```python
from build123d import *

# Parameters (mm, degrees)
F0_R     = 4
F0_R_2   = 29.171031
F1_DEPTH = 10


with BuildPart() as f1:
    # F0 (on Front) → F1 (new body)
    with BuildSketch(Plane.XZ):
        with BuildLine():
            Line((200, 125), (-180, 125))
            ThreePointArc((-180, 125), (-194.142136, 119.142136), (-200, 105))
            Line((-200, 105), (-200, -45))
            ThreePointArc((-200, -45), (-143.431458, -68.431458), (-120, -125))
            Line((-120, -125), (200, -125))
            Line((200, -125), (200, 125))
        make_face()
        with Locations((-55.033423, -4.654916)):
            Circle(F0_R, mode=Mode.SUBTRACT)
        with Locations((5.235739, -4.654916)):
            Circle(F0_R, mode=Mode.SUBTRACT)
        with Locations((66.157822, -4.654916)):
            Circle(F0_R, mode=Mode.SUBTRACT)
        with Locations((118.3732, -4.654916)):
            Circle(F0_R, mode=Mode.SUBTRACT)
        with Locations((160.996102, -4.654916)):
            Circle(F0_R, mode=Mode.SUBTRACT)
        with Locations((-150.960162, 44.787358)):
            Circle(F0_R_2, mode=Mode.SUBTRACT)
        with Locations((-59.337278, 45.036767)):
            Circle(F0_R, mode=Mode.SUBTRACT)
        with Locations((-60.269162, 95.248777)):
            Circle(F0_R, mode=Mode.SUBTRACT)
        with Locations((0.931884, 45.036767)):
            Circle(F0_R, mode=Mode.SUBTRACT)
        with Locations((61.853966, 45.036767)):
            Circle(F0_R, mode=Mode.SUBTRACT)
        with Locations((114.069345, 45.036767)):
            Circle(F0_R, mode=Mode.SUBTRACT)
        with Locations((156.692246, 45.036767)):
            Circle(F0_R, mode=Mode.SUBTRACT)
        with Locations((0, 95.248777)):
            Circle(F0_R, mode=Mode.SUBTRACT)
        with Locations((60.922083, 95.248777)):
            Circle(F0_R, mode=Mode.SUBTRACT)
        with Locations((113.137461, 95.248777)):
            Circle(F0_R, mode=Mode.SUBTRACT)
        with Locations((155.760363, 95.248777)):
            Circle(F0_R, mode=Mode.SUBTRACT)
    extrude(amount=F1_DEPTH)


solid = f1.part
```
Check sheet for the modelled part. Datum: model origin and axes. Units: mm. Round coordinates to 2 decimals unless told otherwise and drop trailing zeros. Order: outer loops, then holes, each group sorted by start corner. A loop starts at its lowest first (then second) coordinate and runs counter-clockwise, first axis right, second up. Notation, with made-up numbers: (-27.75, 14) -> (25.25, 14) arc R25 ccw to (25.25, 46) -> close; hole circle Ø1 at (-22, 41.5). An arc over 180 degrees is marked (long way). One line per item, written item: value. Start each with the question number.
Q1. Cross-section at A-A (x = -130.5). Record the boundary of the cut face in (y, z).
Q2. Mould release check, pull along X, two halves, no side actions. Record for faces 1 (the face through (-3, -10, 2)), 2 (the face through (9.05, -4.93, -3.45)), 3 (the face through (-200, -5, 31)): pulls with the +X half, pulls with the -X half, needs draft (parallel to the pull), parting line crosses it, or undercut.
Q3. Cross-section at B-B (y = -6.75). Give the number of separate pieces and of enclosed holes in the cut face, and give its area (3 significant figures).
Q4. Thickness scan on line 1 (X direction, y = -4.25, z = 97.5); line 2 (X direction, y = -1, z = -8); line 3 (Z direction, x = -172, y = -8). Record the ranges inside material, lowest first.
Completed:
1. outline: (-10, -85.38) -> (0, -85.38) -> (0, 23.99) -> (-10, 23.99) -> close; (-10, 65.58) -> (0, 65.58) -> (0, 125) -> (-10, 125) -> close
2. face 1: needs draft
2. face 2: undercut
2. face 3: pulls with the -X half
3. separate pieces: 1
3. enclosed holes: 16
3. area: 91,500 mm²
4. line 1: x = -200 to -63.58, -56.96 to -3.31, 3.31 to 57.62, 64.23 to 109.83, 116.44 to 152.45, 159.07 to 200
4. line 2: x = -200 to -57.23, -52.84 to 3.04, 7.43 to 63.96, 68.35 to 116.18, 120.57 to 158.8, 163.19 to 200
4. line 3: z = -50.06 to 24.58, 64.99 to 125
